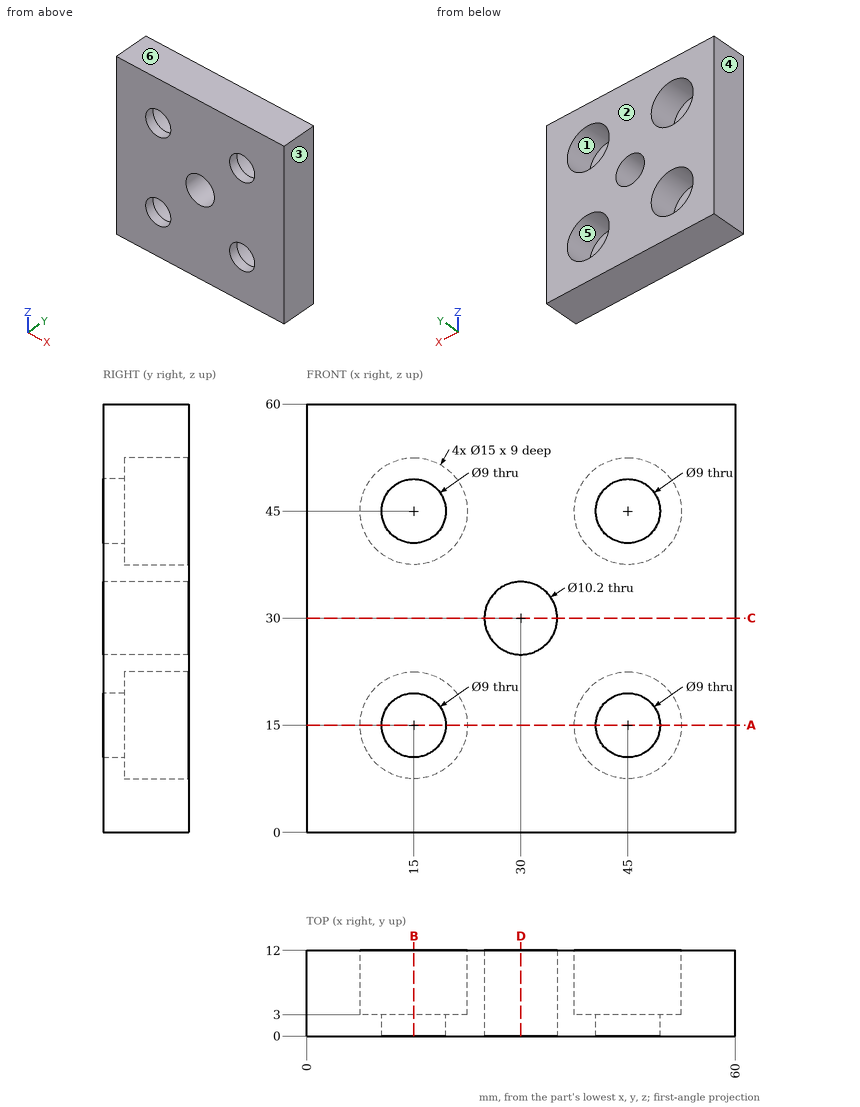
Print and shaded views of the part. All mm, measured from the part's lowest x, y and z. A direction names the side the tool comes from. Coordinates: 2 decimals unless noted, no trailing zeros. Loops run counter-clockwise (first coordinate to the right, second up) from the corner with the lowest first, then second, coordinate; pieces in that order, holes last. Notation, with made-up numbers: (82.25, 81) - (102.25, 81) arc R19 cw to (102.25, 118) - close; hole circle Ø8 at (87.25, -1). An arc over 180 degrees is marked (long way). Use one line per item in the form item = value. Start each with the question number.
1) Band-saw the part on D-D (x = 30). Give the cut face in (y, z), and give its area (3 significant figures).
2) Band-saw the part on B-B (x = 15). Give the cut face in (y, z).
3) Flat gauge pins, fed straight in: pin 1 (8 mm diameter, centred on x = 15, z = 45, fed in from +Y); pin 2 (7.5 mm diameter, centred on x = 13.5, z = 15, fed in from +Y). Where does each tip first touch, or does it go through?
4) Two-plate mould, pull along X, no slides. Class the marked faces 1, 2, 3 and 4: +X half, -X half, draft (parallel to the pull), parting line (faces both ways), or undercut.
5) Band-saw the part on C-C (z = 30). Give the cut face in (x, y).
6) Band-saw the part on A-A (z = 15). Give the cut face in (x, y).
7) Drill centre lines: L1, parallel to X at y = 2, z = 15; L2, parallel to X at y = 9.25, z = 15; L3, parallel to Z at x = 30, y = 2.75. Where is each one in solid material? Low to high. Write a range as from..to.
8) Tool access for the marked faces 5 and 6: list every direction of +Z, -Z, +X, -X, +Y, -Y with a clear straight run to the whole face (end or side of a thin tool).
Check values:
q1.outline = (0, 0) - (12, 0) - (12, 24.9) - (0, 24.9) - close; (0, 35.1) - (12, 35.1) - (12, 60) - (0, 60) - close
q1.area = 598 mm2
q2.outline = (0, 0) - (12, 0) - (12, 7.5) - (3, 7.5) - (3, 10.5) - (0, 10.5) - close; (0, 19.5) - (3, 19.5) - (3, 22.5) - (12, 22.5) - (12, 37.5) - (3, 37.5) - (3, 40.5) - (0, 40.5) - close; (0, 49.5) - (3, 49.5) - (3, 52.5) - (12, 52.5) - (12, 60) - (0, 60) - close
q3.pin_1 = through
q3.pin_2 = 3
q4.face_1 = undercut
q4.face_2 = draft
q4.face_3 = +X half
q4.face_4 = -X half
q5.outline = (0, 0) - (24.9, 0) - (24.9, 12) - (0, 12) - close; (35.1, 0) - (60, 0) - (60, 12) - (35.1, 12) - close
q6.outline = (0, 0) - (10.5, 0) - (10.5, 3) - (7.5, 3) - (7.5, 12) - (0, 12) - close; (19.5, 0) - (40.5, 0) - (40.5, 3) - (37.5, 3) - (37.5, 12) - (22.5, 12) - (22.5, 3) - (19.5, 3) - close; (49.5, 0) - (60, 0) - (60, 12) - (52.5, 12) - (52.5, 3) - (49.5, 3) - close
q7.L1 = 0..10.5, 19.5..40.5, 49.5..60
q7.L2 = 0..7.5, 22.5..37.5, 52.5..60
q7.L3 = 0..24.9, 35.1..60
q8.face_5 = +Y
q8.face_6 = +Z, +X, -X, +Y, -Y
